Design review of the part built by this model. Coordinates are the model's own, in mm. Face numbers are marked on the shaded views. A direction names the side the tool comes from. Coordinates: 2 decimals unless noted, no trailing zeros. Order: outer loops, then holes, each group sorted by start corner. A loop starts at its lowest first (then second) coordinate and runs counter-clockwise, first axis right, second up. Notation, with made-up numbers: M -3,-15.5 L 45,-15.5 A25 cw 45,-1.5 Z; hole C 29.5,83.25 d10. An arc over 180 degrees is marked long. Answer as a JSON object with one key per item and string values.
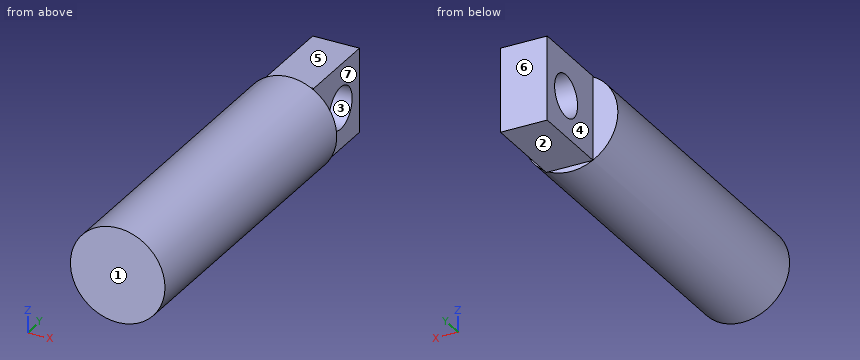
from build123d import *

# Parameters (mm, degrees)
ESQUISSE1_W             = 4.45
ESQUISSE1_H             = 8
BOSS_EXTRU_1_DEPTH      = 8
ESQUISSE2_R             = 4.5
BOSS_EXTRU_2_DEPTH      = 30
ESQUISSE4_R             = 2
ENL_V_MAT_EXTRU_1_DEPTH = 18


with BuildPart() as part:
    # Esquisse1 → Boss.-Extru.1 (new body)
    with BuildSketch(Plane.XY):
        with Locations((0.087605016, -1.300333333)):
            Rectangle(ESQUISSE1_W, ESQUISSE1_H)
    extrude(amount=BOSS_EXTRU_1_DEPTH)

    # Esquisse2 → Boss.-Extru.2 (add)
    with BuildSketch(Plane.XZ.offset(5.300333333)):
        with Locations(Location((0, 3.983435039, 0), (0, 0, 63.197988835))):
            Circle(ESQUISSE2_R)
    extrude(amount=BOSS_EXTRU_2_DEPTH)

    # Esquisse4 → Enlèv. mat.-Extru.1 (cut)
    with BuildSketch(Plane(origin=(2.312605016, 0, 0), x_dir=(0, 0, -1), z_dir=(1, 0, 0))):
        with Locations(Location((-3.87570667, -0.589342017, 0), (0, 0, 90))):
            Circle(ESQUISSE4_R)
    extrude(amount=-ENL_V_MAT_EXTRU_1_DEPTH, mode=Mode.SUBTRACT)


solid = part.part
1) Insertion check: pin 1 Ø3 at (y, z) = (-15, 3.5) entering from -X; pin 2 Ø5 at (y, z) = (-15.5, 7.5) entering from +X; pin 3 Ø3 at (y, z) = (-0.59, 3.88) entering from +X; pin 4 Ø0.5 at (x, z) = (0.5, 8.5) entering from +Y. Each pin has a flat end and moves straight along its axis. Give the tip position at first contact, or say it passes through.
Taken from the geometry:
{"pin 1": "stops at x = -4.5", "pin 2": "stops at x = 4.38", "pin 3": "passes through", "pin 4": "stops at y = -5.3"}
2) Add section D-D (z = 7.5). State the section outline as (x, y) points, and give its area (3 significant figures).
Taken from the geometry:
{"outline": "M -2.81,-35.3 L 2.81,-35.3 L 2.81,-5.3 L 2.31,-5.3 L 2.31,2.7 L -2.14,2.7 L -2.14,-5.3 L -2.81,-5.3 Z", "area": "204 mm2"}
3) Add section C-C (y = 0). State the section outline as (x, z) points.
Taken from the geometry:
{"outline": "M -2.14,0 L 2.31,0 L 2.31,1.96 L -2.14,1.96 Z; M -2.14,5.79 L 2.31,5.79 L 2.31,8 L -2.14,8 Z"}
4) Add section A-A (z = 3.25). State the section outline as (x, y) points.
Taken from the geometry:
{"outline": "M -4.44,-35.3 L 4.44,-35.3 L 4.44,-5.3 L 2.31,-5.3 L 2.31,-2.49 L -2.14,-2.49 L -2.14,-5.3 L -4.44,-5.3 Z; M -2.14,1.31 L 2.31,1.31 L 2.31,2.7 L -2.14,2.7 Z"}
5) Add section B-B (x = -1). State the section outline as (y, z) points, and give its area (3 significant figures).
Taken from the geometry:
{"outline": "M -35.3,-0.4 L -5.3,-0.4 L -5.3,0 L 2.7,0 L 2.7,8 L -5.3,8 L -5.3,8.37 L -35.3,8.37 Z; hole C -0.59,3.88 d4", "area": "315 mm2"}
6) To check wall thickness, follow L1, parallel to Y at x = 0, z = 3.75; L2, parallel to Y at x = 3.25, z = 6.5; L3, parallel to X at y = -22.5, z = 0. State the ranges of each line that lie inside material, in increasing order.
Taken from the geometry:
{"L1": "y = -35.3 to -2.59, 1.41 to 2.7", "L2": "y = -35.3 to -5.3", "L3": "x = -2.09 to 2.09"}
7) Tool access review of the marked faces 4, 5, 6 and 7: name each direction out of +Z, -Z, +X, -X, +Y, -Y from which nothing blocks a thin tool from reaching the whole face with its end or side.
Taken from the geometry:
{"face 4": "+Z, -Z, -X, +Y", "face 5": "+Z, +X, -X, +Y", "face 6": "+Z, -Z, +X, -X, +Y", "face 7": "+Z, -Z, +X, +Y"}
8) Mouldability with a two-part tool opening along Y and no side actions: class the marked faces 1, 2 and 3 as released by +Y, released by -Y, zero draft, split by the parting line, or undercut.
Taken from the geometry:
{"face 1": "released by -Y", "face 2": "zero draft", "face 3": "undercut"}
